```python
from build123d import *

# Parameters (mm, degrees)
SKETCH1_W           = 160
SKETCH1_H           = 15
BOSS_EXTRUDE1_DEPTH = 15
SKETCH2_R           = 1.25
CUT_EXTRUDE1_DEPTH  = 162.400123916
SKETCH3_R           = 1.145
SKETCH3_R_2         = 1.25
CUT_EXTRUDE2_DEPTH  = 162.400123916
SKETCH6_R           = 1.25
CUT_EXTRUDE5_DEPTH  = 10
CUT_EXTRUDE6_START  = -10
SKETCH7_R           = 1.25
CUT_EXTRUDE6_DEPTH  = 10


with BuildPart() as part:
    # Sketch1 → Boss-Extrude1 (new body)
    with BuildSketch(Plane.XY):
        with Locations((80, 7.5)):
            Rectangle(SKETCH1_W, SKETCH1_H)
    extrude(amount=BOSS_EXTRUDE1_DEPTH)

    # Sketch2 → Cut-Extrude1 (cut, through all)
    with BuildSketch(Plane.XY.offset(15)):
        with Locations((40, 7.5)):
            Circle(SKETCH2_R)
        with Locations((120, 7.5)):
            Circle(SKETCH2_R)
    extrude(amount=-CUT_EXTRUDE1_DEPTH, mode=Mode.SUBTRACT)

    # Sketch3 → Cut-Extrude2 (cut, through all)
    with BuildSketch(Plane(origin=(0, 15, 0), x_dir=(1, 0, 0), z_dir=(0, 1, 0))):
        with Locations(Location((40, -7.5, 0), (0, 0, 270))):
            Circle(SKETCH3_R)
        with Locations(Location((120, -7.5, 0), (0, 0, 270))):
            Circle(SKETCH3_R_2)
    extrude(amount=-CUT_EXTRUDE2_DEPTH, mode=Mode.SUBTRACT)

    # Sketch6 → Cut-Extrude5 (cut)
    with BuildSketch(Plane.ZY):
        with Locations((4, 11)):
            Circle(SKETCH6_R)
        with Locations((11, 4)):
            Circle(SKETCH6_R)
    extrude(amount=-CUT_EXTRUDE5_DEPTH, mode=Mode.SUBTRACT)

    # Sketch7 → Cut-Extrude6 (cut)
    with BuildSketch(Plane(origin=(160, 0, 0), x_dir=(0, 0, -1), z_dir=(1, 0, 0)).offset(CUT_EXTRUDE6_START)):
        with Locations(Location((-4, 11, 0), (0, 0, 180))):
            Circle(SKETCH7_R)
        with Locations(Location((-11, 4, 0), (0, 0, 180))):
            Circle(SKETCH7_R)
    extrude(amount=CUT_EXTRUDE6_DEPTH, mode=Mode.SUBTRACT)


solid = part.part
```
Model file for the job. Use its own axes, mm. A direction names the side the tool comes from. Coordinates: 2 decimals unless noted, no trailing zeros. Answer as a JSON object with one key per item and string values. Group by question number.
1) Drill centre lines: L1, parallel to X at y = 5.5, z = 7.75; L2, parallel to Y at x = 157.5, z = 4; L3, parallel to Z at x = 40, y = 11.75 (3 decimals). Where is each one in solid material? Low to high.
2) Pull direction Y, two halves, no side cores. Call faces 4 (the face through (150, 11, 4)), 5 (the face through (79, 0, 7)), 6 (the face through (79, 15, 7)), 7 (the face through (160, 7, 7)): +Y half, -Y half, draft (parallel to the pull), parting line (faces both ways), or undercut.
3) Which spindle directions (+Z, -Z, +X, -X, +Y, -Y) get a long thin tool onto all of the face, cutting with end or side? Do faces 1 (the face through (10, 4, 11)), 2 (the face through (118.75, 7.55, 2.97)), 3 (the face through (154.93, 4.76, 10.01)). Say none if no direction does.
4) Flat gauge pins, fed straight in: pin 1 (2 mm diameter, centred on x = 120, y = 7.5, fed in from +Z); pin 2 (0.8 mm diameter, centred on y = 4.5, z = 11, fed in from -X); pin 3 (1.5 mm diameter, centred on y = 11, z = 4, fed in from +X). Where does each tip first touch, or does it go through?
Check values:
{
 "1": {"L1": "x = 0 to 38.88, 41.12 to 118.78, 121.22 to 160", "L2": "y = 0 to 9.75, 12.25 to 15", "L3": "z = 0 to 6.355, 8.645 to 15"},
 "2": {"face 4": "undercut", "face 5": "-Y half", "face 6": "+Y half", "face 7": "draft"},
 "3": {"face 1": "-X", "face 2": "+Z, -Z", "face 3": "+X"},
 "4": {"pin 1": "passes through", "pin 2": "stops at x = 10", "pin 3": "stops at x = 150"}
}
